Answer from the drawing. Dimensions are ordinates in mm from the lowest x, y and z of the part. A direction names the side the tool comes from. Give positions to 0.01 mm unless a question says otherwise; leave off trailing zeros. Write each loop counter-clockwise with the first axis right and the second up, starting at its lowest first coordinate (ties: lowest second). Pieces come first, ordered by that corner, then holes.
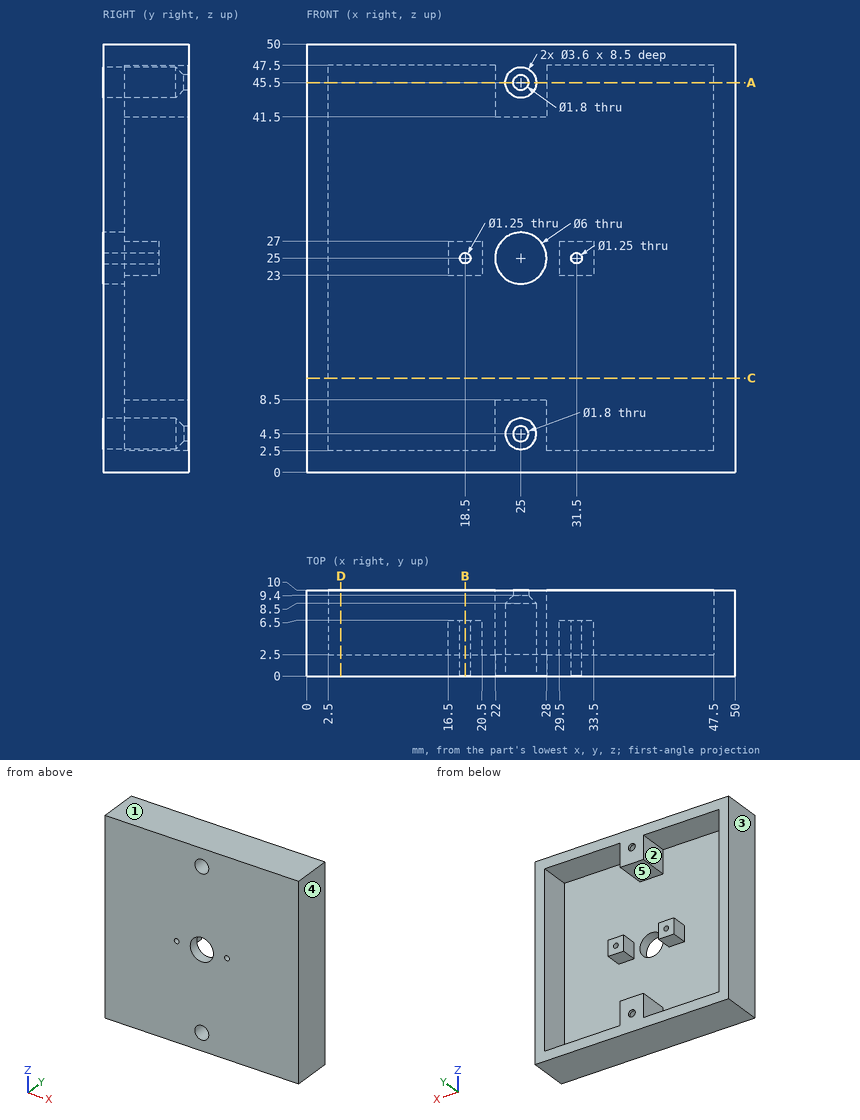
Item 1: Which of the six approach directions +Z, -Z, +X, -X, +Y, -Y give full straight-line access (tool end or side, diameter ignored) to the marked faces 4 and 5?
Conclusion:
face 4: +Z, -Z, +X, +Y, -Y
face 5: +Y
Item 2: A cutting plane is placed at D-D, the plane x = 4. Give the vertices of the cut face in (y, z), plus the area to 4 significant figures.
Conclusion:
outline: (0, 0) - (10, 0) - (10, 2.5) - (2.5, 2.5) - (2.5, 47.5) - (10, 47.5) - (10, 50) - (0, 50) - close
area: 162.5 mm2
Item 3: Consider probe 1 along Z at (x, y) = (25, 9.7); probe 2 along Z at (x, y) = (31.5, 3) (3 decimals); probe 3 along X at (y, z) = (9.55, 45.5). Determine where each line is inside the solid, lowest interval first.
Conclusion:
probe 1: z = 0 to 3.6, 5.4 to 8.5, 41.5 to 44.6, 46.4 to 50
probe 2: z = 0 to 2.5, 23 to 24.375, 25.625 to 27, 47.5 to 50
probe 3: x = 0 to 2.5, 22 to 24.1, 25.9 to 28, 47.5 to 50
Item 4: A cutting plane is placed at A-A, the plane z = 45.5. Give the vertices of the cut face in (x, y).
Conclusion:
outline: (0, 0) - (23.2, 0) - (23.2, 8.5) - (24.1, 9.4) - (24.1, 10) - (22, 10) - (22, 2.5) - (2.5, 2.5) - (2.5, 10) - (0, 10) - close; (25.9, 9.4) - (26.8, 8.5) - (26.8, 0) - (50, 0) - (50, 10) - (47.5, 10) - (47.5, 2.5) - (28, 2.5) - (28, 10) - (25.9, 10) - close
Item 5: Each of these flat-tipped pins is pushed along its axis until it touches: P1, Ø6, axis at x = 10, y = 8, coming from the -Z side; P2, Ø4, axis at x = 38.5, z = 33.5, coming from the +Y side; P3, Ø2, axis at x = 25, z = 4.5, coming from the -Y side. Where does it stop, or does it pass through?
Conclusion:
P1: stops at z = 0
P2: stops at y = 2.5
P3: stops at y = 9.3
Item 6: Determine the mould class of the marked faces 1, 2 and 3 for opening direction X: pulls with the +X half, pulls with the -X half, needs draft (parallel to the pull), parting line crosses it, or undercut.
Conclusion:
face 1: needs draft
face 2: undercut
face 3: pulls with the -X half
Item 7: A cutting plane is placed at C-C, the plane z = 11. Give the vertices of the cut face in (x, y).
Conclusion:
outline: (0, 0) - (50, 0) - (50, 10) - (47.5, 10) - (47.5, 2.5) - (2.5, 2.5) - (2.5, 10) - (0, 10) - close
Item 8: A cutting plane is placed at B-B, the plane x = 18.5. Give the vertices of the cut face in (y, z) (3 decimals), plus the area to 3 significant figures.
Conclusion:
outline: (0, 0) - (10, 0) - (10, 2.5) - (2.5, 2.5) - (2.5, 23) - (6.5, 23) - (6.5, 24.375) - (0, 24.375) - close; (0, 25.625) - (6.5, 25.625) - (6.5, 27) - (2.5, 27) - (2.5, 47.5) - (10, 47.5) - (10, 50) - (0, 50) - close
area: 170 mm2
